Could you check a few things on this model? Use its own coordinates, in mm. Face numbers are marked on the shaded views. A direction names the side the tool comes from. Round coordinates to 2 decimals unless told otherwise and drop trailing zeros. Loops run counter-clockwise (first coordinate to the right, second up) from the corner with the lowest first, then second, coordinate; pieces in that order, holes last. Notation, with made-up numbers: (62.25, 88.25) - (92.25, 88.25) arc R32 cw to (92.25, 115.25) - close; hole circle Ø11 at (28.25, 28.25). An arc over 180 degrees is marked (long way). Answer as CSV lines item,"result". Start each with the question number.
1) I'm going to push flat-ended pins straight in: pin 1 Ø0.8 at (x, y) = (33.5, 6) entering from +Z; pin 2 Ø4 at (x, z) = (35.5, 1) entering from -Y; pin 3 Ø2 at (x, z) = (34, -4) entering from +Y. Where does each tip first touch, or does it pass through?
2) Suppose I cut it at A-A, the plane x = -36.5. Write out the boundary of the cut face in (y, z).
3) Which directions (+Z, -Z, +X, -X, +Y, -Y) give clear straight access to the entire face, cutting with the end or side of a thin tool? Please do the marked faces 1, 2 and 3.
4) Please list where these lines run through material, in increasing order: line 1 along X through (y, z) = (-4, -7.25); line 2 along X through (y, z) = (4.25, -1); line 3 along X through (y, z) = (3.75, -5.75).
```python
from build123d import *

# Parameters (mm, degrees)
SKETCH2_W          = 4
SKETCH2_H          = 2.5
CUT_EXTRUDE1_DEPTH = 8
SKETCH3_W          = 5
SKETCH3_H          = 3
CUT_EXTRUDE2_DEPTH = 6


with BuildPart() as part:
    # Sketch1 → Revolve1 (revolve)
    with BuildSketch(Plane.XY):
        Polygon((-52.05, 0), (52.05, 0), (52.05, 7.5), (50.95, 7.5), (50.95, 7.15), (49.85, 7.15), (49.85, 7.5), (31.85, 7.5), (31.85, 8.5), (16.95, 8.5), (16.95, 8.1), (15.85, 8.1), (15.85, 8.5), (3.85, 8.5), (3.85, 10), (-4.15, 10), (-4.15, 8.5), (-16.15, 8.5), (-16.15, 8.1), (-17.25, 8.1), (-17.25, 8.5), (-32.15, 8.5), (-32.15, 6), (-50.15, 6), (-50.15, 5.75), (-51.25, 5.75), (-51.25, 6), (-52.05, 6), align=None)
    revolve(axis=Axis((-52.05, 0, 0), (1, 0, 0)))

    # Sketch2 → Cut-Extrude1 (cut)
    with BuildSketch(Plane.ZY.offset(32.15)):
        with Locations((0, 4.75)):
            Rectangle(SKETCH2_W, SKETCH2_H)
    extrude(amount=CUT_EXTRUDE1_DEPTH, mode=Mode.SUBTRACT)

    # Sketch3 → Cut-Extrude2 (cut)
    with BuildSketch(Plane(origin=(31.85, 0, 0), x_dir=(0, 0, -1), z_dir=(1, 0, 0))):
        with Locations((0, 6)):
            Rectangle(SKETCH3_W, SKETCH3_H)
    extrude(amount=CUT_EXTRUDE2_DEPTH, mode=Mode.SUBTRACT)


solid = part.part
```
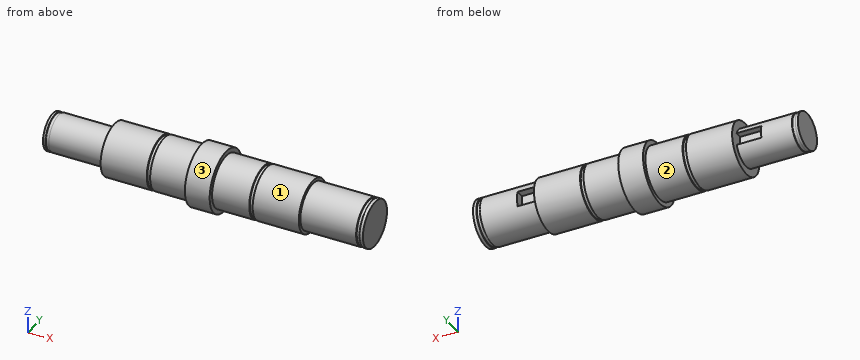
Filled sheet:
1,pin 1,"z = 4.99"
1,pin 2,"y = -7.5"
1,pin 3,"y = 6.87"
2,outline,"(3.5, -2) - (3.5, 2) - (5.66, 2) arc R6 ccw (long way) to (5.66, -2) - close"
3,face 1,"+X"
3,face 2,"-X"
3,face 3,"+X, -X"
4,line 1,"-32.15 to -17.25, -16.15 to 15.85, 16.95 to 31.85"
4,line 2,"-52.05 to -40.15, -32.15 to 52.05"
4,line 3,"-32.15 to 52.05"
